```python
from build123d import *

# Parameters (mm, degrees)
BOSS_EXTRUDE1_DEPTH = 25
SKETCH3_R           = 2
CUT_EXTRUDE1_DEPTH  = 21.5000001
SKETCH4_R           = 2
CUT_EXTRUDE2_DEPTH  = 21.5000001
CUT_EXTRUDE3_START  = -1.6
CUT_EXTRUDE3_DEPTH  = 19.9000001
CUT_EXTRUDE4_START  = -1.6
CUT_EXTRUDE4_DEPTH  = 19.9000001
CHAMFER1_SIZE       = 7


with BuildPart() as part:
    # Sketch1 → Boss-Extrude1 (new body)
    with BuildSketch(Plane(origin=(0, 0, 0), x_dir=(1, 0, 0), z_dir=(0, 1, 0))):
        with BuildLine():
            Line((0, 0), (0, 25))
            Line((0, 25), (4, 25))
            Line((4, 25), (4, 10))
            ThreePointArc((4, 10), (5.757359313, 5.757359313), (10, 4))
            Line((10, 4), (25, 4))
            Line((25, 4), (25, 0))
            Line((25, 0), (0, 0))
        make_face()
    extrude(amount=BOSS_EXTRUDE1_DEPTH)

    # Sketch2 → Cut-Revolve2 (revolve, cut)
    with BuildSketch(Plane.XY):
        with BuildLine():
            Line((8, 0), (0, 0))
            Line((0, 0), (0, -0.947269394))
            Line((0, -0.947269394), (27.823952472, -0.947269394))
            Line((27.823952472, -0.947269394), (27.823952472, 28.581077379))
            Line((27.823952472, 28.581077379), (0, 28.581077379))
            Line((0, 28.581077379), (0, 25))
            Line((0, 25), (8, 25))
            ThreePointArc((8, 25), (20.5, 12.5), (8, 0))
        make_face()
    revolve(axis=Axis((0, 25, 0), (0, 1, 0)), mode=Mode.SUBTRACT)

    # Sketch3 → Cut-Extrude1 (cut, through all)
    with BuildSketch(Plane.XY):
        with Locations((12, 12.5)):
            Circle(SKETCH3_R)
    extrude(amount=-CUT_EXTRUDE1_DEPTH, mode=Mode.SUBTRACT)

    # Sketch4 → Cut-Extrude2 (cut, through all)
    with BuildSketch(Plane.ZY):
        with Locations((-12, 12.5)):
            Circle(SKETCH4_R)
    extrude(amount=-CUT_EXTRUDE2_DEPTH, mode=Mode.SUBTRACT)

    # Sketch5 → Cut-Extrude3 (cut, through all)
    with BuildSketch(Plane.ZY.offset(CUT_EXTRUDE3_START)):
        Polygon((-8.4, 14.578460969), (-12, 16.656921938), (-15.6, 14.578460969), (-15.6, 10.421539031), (-12, 8.343078062), (-8.4, 10.421539031), align=None)
    extrude(amount=-CUT_EXTRUDE3_DEPTH, mode=Mode.SUBTRACT)

    # Sketch6 → Cut-Extrude4 (cut, through all)
    with BuildSketch(Plane.XY.offset(CUT_EXTRUDE4_START)):
        Polygon((12, 8.343078062), (15.6, 10.421539031), (15.6, 14.578460969), (12, 16.656921938), (8.4, 14.578460969), (8.4, 10.421539031), align=None)
    extrude(amount=-CUT_EXTRUDE4_DEPTH, mode=Mode.SUBTRACT)

    # Chamfer1
    chamfer1_edges = [part.edges().sort_by_distance(p)[0] for p in [
        (0, 12.5, 0),
    ]]
    chamfer(chamfer1_edges, length=CHAMFER1_SIZE)


solid = part.part
```
Source: CAD feature listing. Evaluate the final solid. Frame: model axes, mm. A direction names the side the tool comes from. Round coordinates to 2 decimals unless told otherwise and drop trailing zeros. Use CSV: the item, a comma, the result in double quotes.
(1) Access query for faces 1 (the face through (0, 12, -15)), 2 (the face through (16, 12, -4)), 3 (the face through (2.783, 15.632, -13.775)), 4 (the face through (10.17, 9.4, -2.89)). Directions: +Z, -Z, +X, -X, +Y, -Y. A direction counts if a zero-diameter tool reaches every point of the face in a straight line with its end or side. Return the directions, or none.
Report:
face 1,"+Z, -Z, -X, +Y, -Y"
face 2,"-Z, +X, +Y, -Y"
face 3,"+X"
face 4,"-Z"
(2) First-contact query: pin 1 Ø1.3 at (x, y) = (3.5, 12.5) entering from -Z; pin 2 Ø8 at (y, z) = (17.5, -17) entering from +X; pin 3 Ø1.9 at (y, z) = (12, -2.5) entering from -X. Flat tips, straight axial feed; report the tip coordinate or a pass-through.
Report:
pin 1,"z = -20.3"
pin 2,"x = 4"
pin 3,"x = 3.55"
(3) Section A-A on y = 12.5. Count the separate pieces of the cut face and the enclosed holes in it, and give its area (3 significant figures).
Report:
separate pieces,"3"
enclosed holes,"0"
area,"82.6 mm^2"
(4) Ray query, L1, parallel to Z at x = 19.5, y = 10.5; L2, parallel to Y at x = 1.75, z = -11; L3, parallel to X at y = 19.75, z = -10. Return the intervals inside material, ascending.
Report:
L1,"-4 to 0"
L2,"0.4 to 8.92, 16.08 to 24.6"
L3,"0 to 4"
(5) Pull-direction query (X, two-part tool) for faces 5 (the face through (4, 12, -16)), 6 (the face through (13.775, 9.368, -2.783)), 7 (the face through (2.78, 9.4, -13.83)), 8 (the face through (15.6, 12, -3)); classes: +X half, -X half, draft (parallel to the pull), parting line (faces both ways), or undercut.
Report:
face 5,"+X half"
face 6,"undercut"
face 7,"draft"
face 8,"undercut"
